Read the model definition and answer for the solid it produces. Units are mm, in the model's axes. A direction names the side the tool comes from. Round coordinates to 2 decimals unless told otherwise and drop trailing zeros. Order: outer loops, then holes, each group sorted by start corner. A loop starts at its lowest first (then second) coordinate and runs counter-clockwise, first axis right, second up.
from build123d import *

# Parameters (mm, degrees)
BOXSIDE_DEPTH      = 6.35
SKETCH2_R          = 3.96875
CUT_EXTRUDE1_DEPTH = 99.986703653


with BuildPart() as part:
    # Sketch1 → BOXSIDE (new body)
    with BuildSketch(Plane.XY):
        Polygon((-63.5, 38.1), (-63.5, 63.5), (63.5, 63.5), (63.5, 38.1), (69.85, 38.1), (69.85, 12.7), (63.5, 12.7), (63.5, -12.7), (69.85, -12.7), (69.85, -38.1), (63.5, -38.1), (63.5, -63.5), (44.45, -63.5), (44.45, -69.85), (25.4, -69.85), (25.4, -63.5), (-25.4, -63.5), (-25.4, -69.85), (-44.45, -69.85), (-44.45, -63.5), (-63.5, -63.5), (-63.5, -38.1), (-57.15, -38.1), (-57.15, -12.7), (-63.5, -12.7), (-63.5, 12.7), (-57.15, 12.7), (-57.15, 38.1), align=None)
    extrude(amount=BOXSIDE_DEPTH)

    # Sketch2 → Cut-Extrude1 (cut, through all)
    with BuildSketch(Plane.XY.offset(6.35)):
        with Locations((3.175, 0)):
            Circle(SKETCH2_R)
        with Locations((38.1, 5.339056325)):
            Circle(SKETCH2_R)
        with Locations((17.105250883, 25.77544668)):
            Circle(SKETCH2_R)
    extrude(amount=-CUT_EXTRUDE1_DEPTH, mode=Mode.SUBTRACT)


solid = part.part
Q1. A cutting plane is placed at C-C, the plane x = -6.5. Give the vertices of the cut face in (y, z).
Outcome:
outline: (-63.5, 0) - (63.5, 0) - (63.5, 6.35) - (-63.5, 6.35) - close
Q2. For faces 5 (the face through (67, 12.7, 3)), 6 (the face through (0, -63.5, 3)), 7 (the face through (67, 38.1, 3)), determine the directions among +Z, -Z, +X, -X, +Y, -Y from which every point of the face is accessible in a straight line to the end or side of a thin tool.
Outcome:
face 5: +Z, -Z, +X
face 6: +Z, -Z, -Y
face 7: +Z, -Z, +X, +Y
Q3. Straight lines are drawn through the part: probe 1 along X at (y, z) = (5, 0.5); probe 2 along X at (y, z) = (-9, 5). For each, find the intervals that lie inside material, in ascending order.
Outcome:
probe 1: x = -63.5 to 34.15, 42.05 to 63.5
probe 2: x = -63.5 to 63.5
Q4. A cutting plane is placed at B-B, the plane z = 2. Give the number of separate pieces and of enclosed holes in the cut face, plus the area to 3 significant figures.
Outcome:
separate pieces: 1
enclosed holes: 3
area: 16,200 mm2
Q5. Flat-ended cylindrical pins translate along their axes: pin 1 (9 mm diameter, centred on x = 38.1, y = 5.34, fed in from -Z); pin 2 (3 mm diameter, centred on y = -26.5, z = 4.5, fed in from -X); pin 3 (1.9 mm diameter, centred on y = 50.5, z = 2.5, fed in from +X); pin 4 (1.9 mm diameter, centred on y = -67, z = 3, fed in from +X). Find the tip coordinate at first contact, or state that the pin passes through.
Outcome:
pin 1: stops at z = 0
pin 2: stops at x = -57.15
pin 3: stops at x = 63.5
pin 4: stops at x = 44.45
Q6. A cutting plane is placed at A-A, the plane x = 38.1. Give the vertices of the cut face in (y, z), plus the area to 3 significant figures.
Outcome:
outline: (-69.85, 0) - (1.37, 0) - (1.37, 6.35) - (-69.85, 6.35) - close; (9.31, 0) - (63.5, 0) - (63.5, 6.35) - (9.31, 6.35) - close
area: 796 mm2
Q7. For a pull along X with two mould halves and no side action, classify faces 1 (the face through (69.85, -25, 3)), 2 (the face through (34.951, 2.924, 3.219)), 3 (the face through (-63.5, 51, 3)), 4 (the face through (35, -69.85, 3)) as released by +X, released by -X, zero draft, split by the parting line, or undercut.
Outcome:
face 1: released by +X
face 2: undercut
face 3: released by -X
face 4: zero draft
